```python
from build123d import *

# Parameters (mm, degrees)
SKETCH1_W           = 30
SKETCH1_H           = 26
BOSS_EXTRUDE1_DEPTH = 30
SKETCH2_R           = 5.25
CUT_EXTRUDE1_DEPTH  = 15
CUT_EXTRUDE2_REACH  = 37.972
SKETCH3_R           = 2.6
SKETCH4_R           = 2.65
BOSS_EXTRUDE2_DEPTH = 6
CHAMFER1_SIZE       = 8
CHAMFER1_SIZE2      = 13.856406461
SKETCH5_W           = 10
SKETCH5_H           = 20
CUT_EXTRUDE3_DEPTH  = 20
CHAMFER2_SIZE       = 2
SKETCH6_W           = 14
SKETCH6_H           = 8
SKETCH6_R           = 1.95
BOSS_EXTRUDE3_DEPTH = 8
CHAMFER3_SIZE       = 5
CHAMFER3_SIZE2      = 7.140740034


with BuildPart() as part:
    # Sketch1 → Boss-Extrude1 (new body)
    with BuildSketch(Plane.XY):
        Rectangle(SKETCH1_W, SKETCH1_H)
    extrude(amount=BOSS_EXTRUDE1_DEPTH)

    # Sketch2 → Cut-Extrude1 (cut)
    with BuildSketch(Plane.XY):
        with Locations((0, 5)):
            Circle(SKETCH2_R)
    extrude(amount=CUT_EXTRUDE1_DEPTH, mode=Mode.SUBTRACT)

    # Sketch3 → Cut-Extrude2 (cut, up to next)
    with BuildSketch(Plane.XY, mode=Mode.PRIVATE) as cut_extrude2_sk1:
        with Locations((0, 4.5)):
            Circle(SKETCH3_R)
    cut_extrude2_tool1 = extrude(cut_extrude2_sk1.sketch, amount=CUT_EXTRUDE2_REACH, mode=Mode.PRIVATE) & part.part
    add(cut_extrude2_tool1.solids().sort_by_distance((0, 4.5, 0))[0], mode=Mode.SUBTRACT)

    # Sketch4 → Boss-Extrude2 (add)
    # profile 1 of 2: a face of its own
    with BuildSketch(Plane.XZ.offset(13)):
        with BuildLine():
            Line((-15, 30), (-27.472160356, 14.365256125))
            ThreePointArc((-27.472160356, 14.365256125), (-28.738776961, 8.10556471), (-24.395973154, 3.422818792))
            Line((-24.395973154, 3.422818792), (-15, 0))
            Line((-15, 0), (-15, 30))
        make_face()
        with Locations(Location((-22, 10, 0), (0, 0, 270))):
            Circle(SKETCH4_R, mode=Mode.SUBTRACT)
    # profile 2 of 2: a face of its own
    with BuildSketch(Plane.XZ.offset(13)):
        with BuildLine():
            Line((15, 0), (24.395973154, 3.422818792))
            ThreePointArc((24.395973154, 3.422818792), (28.738776961, 8.10556471), (27.472160356, 14.365256125))
            Line((27.472160356, 14.365256125), (15, 30))
            Line((15, 30), (15, 0))
        make_face()
        with Locations(Location((22, 10, 0), (0, 0, 90))):
            Circle(SKETCH4_R, mode=Mode.SUBTRACT)
    extrude(amount=-BOSS_EXTRUDE2_DEPTH)

    # Chamfer1
    chamfer1_edges = [part.edges().sort_by_distance(p)[0] for p in [
        (-15, 13, 15),
        (15, 13, 15),
    ]]
    chamfer1_side = [part.faces().sort_by_distance(p)[0] for p in [
        (0, 13, 15),
    ]]
    chamfer(chamfer1_edges, length=CHAMFER1_SIZE, length2=CHAMFER1_SIZE2, reference=chamfer1_side[0])

    # Sketch5 → Cut-Extrude3 (cut, symmetric)
    with BuildSketch(Plane(origin=(0, 0, 0), x_dir=(0, 0, -1), z_dir=(1, 0, 0))):
        with Locations((-5, 3)):
            Rectangle(SKETCH5_W, SKETCH5_H)
    extrude(amount=CUT_EXTRUDE3_DEPTH, both=True, mode=Mode.SUBTRACT)

    # Chamfer2
    chamfer2_edges = [part.edges().sort_by_distance(p)[0] for p in [
        (-15, -7, 20),
        (15, -7, 20),
        (0, -7, 10),
    ]]
    chamfer(chamfer2_edges, length=CHAMFER2_SIZE)

    # Sketch6 → Boss-Extrude3 (add)
    with BuildSketch(Plane(origin=(0, 0, 10), x_dir=(-1, 0, 0), z_dir=(0, 0, -1))):
        with Locations((0, 17)):
            Rectangle(SKETCH6_W, SKETCH6_H)
        with Locations((0, 17)):
            Circle(SKETCH6_R, mode=Mode.SUBTRACT)
    extrude(amount=-BOSS_EXTRUDE3_DEPTH)

    # Chamfer3
    chamfer3_edges = [part.edges().sort_by_distance(p)[0] for p in [
        (7, 21, 14),
        (-7, 21, 14),
    ]]
    chamfer3_side = [part.faces().sort_by_distance(p)[0] for p in [
        (0, 21, 14),
    ]]
    chamfer(chamfer3_edges, length=CHAMFER3_SIZE, length2=CHAMFER3_SIZE2, reference=chamfer3_side[0])


solid = part.part
```
Model file for the job. Use its own axes, mm. A direction names the side the tool comes from. Give positions to 0.01 mm unless a question says otherwise; leave off trailing zeros. Order: outer loops, then holes, each group sorted by start corner. A loop starts at its lowest first (then second) coordinate and runs counter-clockwise, first axis right, second up.
1) Wall check: probe 1 along X at (y, z) = (-9.25, 10); probe 2 along Y at (x, z) = (0, 22.5); probe 3 along Y at (x, z) = (-17, 20.5). Give the ranges that are in metal, low to high.
2) 3-axis set-ups, long thin cutter, end or side, ignore diameter. For faces 1 (the flat face through (-0.1, 7.4, 15)), 2 (the cylindrical face through (0.423, 15.096, 13.944)), 3 (the flat face through (-15, -3, 20)), 4 (the flat face through (-0.4, -7, 7.8)), 5 (the flat face through (0.2, -0.5, 10)): which of +Z, -Z, +X, -X, +Y, -Y reach the whole face in a straight line?
3) Saw through at B-B, the plane y = -11. Write the cut outline in (x, z).
4) Pin check, flat tips, straight feed: pin 1 (5 mm diameter, centred on y = -3, z = 12, fed in from +X); pin 2 (8.5 mm diameter, centred on x = -2, y = 3, fed in from -Z); pin 3 (5 mm diameter, centred on y = -0.5, z = 15.5, fed in from +X). Stop position of each tip, or through.
5) Saw through at C-C, the plane y = 17. Write the cut outline in (x, z), then the cut area to 3 significant figures.
6) Saw through at A-A, the plane x = 0. Write the cut outline in (y, z), then the cut area to 3 significant figures.
7) Saw through at D-D, the plane x = 22. Write the cut outline in (y, z) (3 decimals).
8) Mould opens along Y. For faces 6 (the cylindrical face through (-0.338, 7.078, 22.395)), 7 (the cylindrical face through (-21.883, -10.042, 12.647)), 8 (the flat face through (-16, -6, 19)) say: +Y half, -Y half, draft (parallel to the pull), parting line (faces both ways), or undercut.
Computed:
1. probe 1: x = -29 to -24.65, -19.35 to 19.35, 24.65 to 29
1. probe 2: y = -13 to 1.9, 7.1 to 13
1. probe 3: y = -13 to -7
2. face 1: -Z
2. face 2: +Z, -Z
2. face 3: +Z, -Z, -X, +Y
2. face 4: -Z, +Y
2. face 5: -Z, +X, -X, +Y
3. outline: (-27.47, 14.37) arc R7 ccw to (-24.4, 3.42) - (-15, 0) - (15, 0) - (24.4, 3.42) arc R7 ccw to (27.47, 14.37) - (15, 30) - (-15, 30) - close; hole circle Ø5.3 at (-22, 10); hole circle Ø5.3 at (22, 10)
4. pin 1: stops at x = 15.5
4. pin 2: stops at z = 10
4. pin 3: stops at x = 15
5. outline: (-4.8, 10) - (-1.95, 10) - (-1.95, 18) - (-4.8, 18) - close; (1.95, 10) - (4.8, 10) - (4.8, 18) - (1.95, 18) - close
5. area: 45.6 mm2
6. outline: (-13, 0) - (-7, 0) - (-7, 8) - (-5, 10) - (-0.25, 10) - (-0.25, 15) - (1.9, 15) - (1.9, 30) - (-13, 30) - close; (7.1, 15) - (10.25, 15) - (10.25, 10) - (15.05, 10) - (15.05, 18) - (13, 18) - (13, 30) - (7.1, 30) - close; (18.95, 10) - (21, 10) - (21, 18) - (18.95, 18) - close
6. area: 484 mm2
7. outline: (-13, 2.55) - (-7, 2.55) - (-7, 7.35) - (-13, 7.35) - close; (-13, 12.65) - (-7, 12.65) - (-7, 21.225) - (-13, 21.225) - close
8. face 6: undercut
8. face 7: draft
8. face 8: +Y half
